```python
from build123d import *

# Parameters (mm, degrees)
F1_DEPTH = 5


# Not quite as in the source:
# - a feature names something its author has since deleted; it is built from what else it names


with BuildPart() as f1:
    # F0 (on Top) → F1 (new body)
    with BuildSketch(Plane.XY):
        with BuildLine():
            ThreePointArc((-1, 3.8729833462), (0, 4), (1, 3.8729833462))
            Line((1, 3.8729833462), (0.4997557997, 7.984375))
            Line((0.4997557997, 7.984375), (0, 8))
            Line((0, 8), (-0.4997557997, 7.984375))
            Line((-0.4997557997, 7.984375), (-1, 3.8729833462))
        make_face()
        with BuildLine():
            ThreePointArc((4, 0), (3.9681187851, 0.5040171699), (3.8729833462, 1))
            ThreePointArc((3.8729833462, 1), (3.8637033052, 1.0352761804), (3.8541019662, 1.0704662693))
            ThreePointArc((3.8541019662, 1.0704662693), (3.4641016151, 2), (2.8541019662, 2.8025170769))
            ThreePointArc((2.8541019662, 2.8025170769), (2.8284271247, 2.8284271247), (2.8025170769, 2.8541019662))
            ThreePointArc((2.8025170769, 2.8541019662), (2, 3.4641016151), (1.0704662693, 3.8541019662))
            ThreePointArc((1.0704662693, 3.8541019662), (1.0352761804, 3.8637033052), (1, 3.8729833462))
            ThreePointArc((1, 3.8729833462), (0, 4), (-1, 3.8729833462))
            ThreePointArc((-1, 3.8729833462), (-1.0352761804, 3.8637033052), (-1.0704662693, 3.8541019662))
            ThreePointArc((-1.0704662693, 3.8541019662), (-2, 3.4641016151), (-2.8025170769, 2.8541019662))
            ThreePointArc((-2.8025170769, 2.8541019662), (-2.8284271247, 2.8284271247), (-2.8541019662, 2.8025170769))
            ThreePointArc((-2.8541019662, 2.8025170769), (-3.4641016151, 2), (-3.8541019662, 1.0704662693))
            ThreePointArc((-3.8541019662, 1.0704662693), (-3.8637033052, 1.0352761804), (-3.8729833462, 1))
            ThreePointArc((-3.8729833462, 1), (-4, 0), (-3.8729833462, -1))
            ThreePointArc((-3.8729833462, -1), (-3.8637033052, -1.0352761804), (-3.8541019662, -1.0704662693))
            ThreePointArc((-3.8541019662, -1.0704662693), (-3.4641016151, -2), (-2.8541019662, -2.8025170769))
            ThreePointArc((-2.8541019662, -2.8025170769), (-2.8284271247, -2.8284271247), (-2.8025170769, -2.8541019662))
            ThreePointArc((-2.8025170769, -2.8541019662), (-2, -3.4641016151), (-1.0704662693, -3.8541019662))
            ThreePointArc((-1.0704662693, -3.8541019662), (-1.0352761804, -3.8637033052), (-1, -3.8729833462))
            ThreePointArc((-1, -3.8729833462), (0, -4), (1, -3.8729833462))
            ThreePointArc((1, -3.8729833462), (1.0352761804, -3.8637033052), (1.0704662693, -3.8541019662))
            ThreePointArc((1.0704662693, -3.8541019662), (2, -3.4641016151), (2.8025170769, -2.8541019662))
            ThreePointArc((2.8025170769, -2.8541019662), (2.8284271247, -2.8284271247), (2.8541019662, -2.8025170769))
            ThreePointArc((2.8541019662, -2.8025170769), (3.4641016151, -2), (3.8541019662, -1.0704662693))
            ThreePointArc((3.8541019662, -1.0704662693), (3.8637033052, -1.0352761804), (3.8729833462, -1))
            ThreePointArc((3.8729833462, -1), (3.9681187851, -0.5040171699), (4, 0))
        make_face()
        Polygon((2, 1.1547005384), (2, 0), (2, -1.1547005384), (1.0000000433, -1.7320507826), (0, -2.3094010768), (-1.0000000161, -1.7320507983), (-2, -1.1547005384), (-2, 0), (-2, 1.1547005384), (-1.0000000433, 1.7320507826), (0, 2.3094010768), (0.9999999889, 1.732050814), align=None, mode=Mode.SUBTRACT)
        with BuildLine():
            Line((2.8025170769, 2.8541019662), (4.4249887183, 6.6647936835))
            Line((4.4249887183, 6.6647936835), (4, 6.9282032303))
            Line((4, 6.9282032303), (3.5593862817, 7.1645494832))
            Line((3.5593862817, 7.1645494832), (1.0704662693, 3.8541019662))
            ThreePointArc((1.0704662693, 3.8541019662), (2, 3.4641016151), (2.8025170769, 2.8541019662))
        make_face()
        with BuildLine():
            Line((3.8541019662, 1.0704662693), (7.1645494832, 3.5593862817))
            Line((7.1645494832, 3.5593862817), (6.9282032303, 4))
            Line((6.9282032303, 4), (6.6647936835, 4.4249887183))
            Line((6.6647936835, 4.4249887183), (2.8541019662, 2.8025170769))
            ThreePointArc((2.8541019662, 2.8025170769), (3.4641016151, 2), (3.8541019662, 1.0704662693))
        make_face()
        with BuildLine():
            Line((7.984375, -0.4997557997), (8, 0))
            Line((8, 0), (7.984375, 0.4997557997))
            Line((7.984375, 0.4997557997), (3.8729833462, 1))
            ThreePointArc((3.8729833462, 1), (3.9681187851, 0.5040171699), (4, 0))
            ThreePointArc((4, 0), (3.9681187851, -0.5040171699), (3.8729833462, -1))
            Line((3.8729833462, -1), (7.984375, -0.4997557997))
        make_face()
        with BuildLine():
            Line((6.9282032303, -4), (7.1645494832, -3.5593862817))
            Line((7.1645494832, -3.5593862817), (3.8541019662, -1.0704662693))
            ThreePointArc((3.8541019662, -1.0704662693), (3.4641016151, -2), (2.8541019662, -2.8025170769))
            Line((2.8541019662, -2.8025170769), (6.6647936835, -4.4249887183))
            Line((6.6647936835, -4.4249887183), (6.9282032303, -4))
        make_face()
        with BuildLine():
            Line((4, -6.9282032303), (4.4249887183, -6.6647936835))
            Line((4.4249887183, -6.6647936835), (2.8025170769, -2.8541019662))
            ThreePointArc((2.8025170769, -2.8541019662), (2, -3.4641016151), (1.0704662693, -3.8541019662))
            Line((1.0704662693, -3.8541019662), (3.5593862817, -7.1645494832))
            Line((3.5593862817, -7.1645494832), (4, -6.9282032303))
        make_face()
        with BuildLine():
            Line((0.4997557997, -7.984375), (1, -3.8729833462))
            ThreePointArc((1, -3.8729833462), (0, -4), (-1, -3.8729833462))
            Line((-1, -3.8729833462), (-0.4997557997, -7.984375))
            Line((-0.4997557997, -7.984375), (0, -8))
            Line((0, -8), (0.4997557997, -7.984375))
        make_face()
        with BuildLine():
            Line((-3.5593862817, -7.1645494832), (-1.0704662693, -3.8541019662))
            ThreePointArc((-1.0704662693, -3.8541019662), (-2, -3.4641016151), (-2.8025170769, -2.8541019662))
            Line((-2.8025170769, -2.8541019662), (-4.4249887183, -6.6647936835))
            Line((-4.4249887183, -6.6647936835), (-4, -6.9282032303))
            Line((-4, -6.9282032303), (-3.5593862817, -7.1645494832))
        make_face()
        with BuildLine():
            Line((-6.6647936835, -4.4249887183), (-2.8541019662, -2.8025170769))
            ThreePointArc((-2.8541019662, -2.8025170769), (-3.4641016151, -2), (-3.8541019662, -1.0704662693))
            Line((-3.8541019662, -1.0704662693), (-7.1645494832, -3.5593862817))
            Line((-7.1645494832, -3.5593862817), (-6.9282032303, -4))
            Line((-6.9282032303, -4), (-6.6647936835, -4.4249887183))
        make_face()
        with BuildLine():
            ThreePointArc((-3.8729833462, -1), (-4, 0), (-3.8729833462, 1))
            Line((-3.8729833462, 1), (-7.984375, 0.4997557997))
            Line((-7.984375, 0.4997557997), (-8, 0))
            Line((-8, 0), (-7.984375, -0.4997557997))
            Line((-7.984375, -0.4997557997), (-3.8729833462, -1))
        make_face()
        with BuildLine():
            ThreePointArc((-3.8541019662, 1.0704662693), (-3.4641016151, 2), (-2.8541019662, 2.8025170769))
            Line((-2.8541019662, 2.8025170769), (-6.6647936835, 4.4249887183))
            Line((-6.6647936835, 4.4249887183), (-6.9282032303, 4))
            Line((-6.9282032303, 4), (-7.1645494832, 3.5593862817))
            Line((-7.1645494832, 3.5593862817), (-3.8541019662, 1.0704662693))
        make_face()
        with BuildLine():
            ThreePointArc((-2.8025170769, 2.8541019662), (-2, 3.4641016151), (-1.0704662693, 3.8541019662))
            Line((-1.0704662693, 3.8541019662), (-3.5593862817, 7.1645494832))
            Line((-3.5593862817, 7.1645494832), (-4, 6.9282032303))
            Line((-4, 6.9282032303), (-4.4249887183, 6.6647936835))
            Line((-4.4249887183, 6.6647936835), (-2.8025170769, 2.8541019662))
        make_face()
    extrude(amount=F1_DEPTH)


solid = f1.part
```
Here's how the part is built. I have some questions about the finished solid (model axes, mm). A direction names the side the tool comes from. Coordinates: 2 decimals unless noted, no trailing zeros. Order: outer loops, then holes, each group sorted by start corner. A loop starts at its lowest first (then second) coordinate and runs counter-clockwise, first axis right, second up.
1) We'd pull the mould along X, two halves only. Please class faces 1 (the face through (-5.49, -2.3, 2.46)), 2 (the face through (2, -2, 0)), 3 (the face through (-2.3, 5.49, 2.46)): +X half, -X half, draft (parallel to the pull), parting line (faces both ways), or undercut.
2) Which directions (+Z, -Z, +X, -X, +Y, -Y) give clear straight access to the entire face, cutting with the end or side of a thin tool? Please do faces 4 (the face through (-2, 0, 2)), 5 (the face through (2.33, 5.53, 2.46)), 6 (the face through (2.3, -5.49, 2.46)), 7 (the face through (5.9, -0.753, 2.465)), 8 (the face through (-5.957, -0.746, 2.465)).
3) Imagine slicing it at B-B on x = 0.75. List the corners of the cut face in (y, z) for me, and give its area (3 significant figures).
4) Imagine slicing it at D-D on x = -4.75. List the corners of the cut face in (y, z) for me.
5) Will this pin go through, and if not, where does the flat tip stop? pin 1 (3 mm diameter, centred on x = 6, z = 2, fed in from -Y) (3 decimals).
6) I need wall thicknesses on line 1 (X direction, y = -3, z = 3.3); line 2 (X direction, y = -4.75, z = 0.2); line 3 (Y direction, x = -4.5, z = 3.15). Which ranges of each line are inside material? Lowest first, please.
7) Imagine slicing it at A-A on y = 3.25. List the corners of the cut face in (x, z) for me.
8) Imagine slicing it at C-C on y = 0.75. List the corners of the cut face in (x, z) for me.
Response values:
1. face 1: -X half
1. face 2: draft
1. face 3: undercut
2. face 4: +Z, -Z
2. face 5: +Z, -Z, +Y
2. face 6: +Z, -Z, -Y
2. face 7: +Z, -Z, +X
2. face 8: +Z, -Z, -X
3. outline: (-5.93, 0) - (-1.88, 0) - (-1.88, 5) - (-5.93, 5) - close; (1.88, 0) - (5.93, 0) - (5.93, 5) - (1.88, 5) - close
3. area: 40.5 mm2
4. outline: (-3.61, 0) - (-1.74, 0) - (-1.74, 5) - (-3.61, 5) - close; (-0.89, 0) - (0.89, 0) - (0.89, 5) - (-0.89, 5) - close; (1.74, 0) - (3.61, 0) - (3.61, 5) - (1.74, 5) - close
5. pin 1: stops at y = -4.425
6. line 1: x = -6.42 to -3.32, -2.86 to 2.86, 3.32 to 6.42
6. line 2: x = -3.61 to -1.74, -0.89 to 0.89, 1.74 to 3.61
6. line 3: y = -3.5 to -1.56, -0.92 to 0.92, 1.56 to 3.5
7. outline: (-6.75, 0) - (-3.91, 0) - (-3.91, 5) - (-6.75, 5) - close; (-2.97, 0) - (2.97, 0) - (2.97, 5) - (-2.97, 5) - close; (3.91, 0) - (6.75, 0) - (6.75, 5) - (3.91, 5) - close
8. outline: (-5.93, 0) - (-2, 0) - (-2, 5) - (-5.93, 5) - close; (2, 0) - (5.93, 0) - (5.93, 5) - (2, 5) - close
